Study the drawing (mm; zero at the part's minimum x, y, z) and answer. A direction names the side the tool comes from. Round coordinates to 2 decimals unless told otherwise and drop trailing zeros. Write each loop counter-clockwise with the first axis right and the second up, starting at its lowest first coordinate (ties: lowest second). Pieces come first, ordered by that corner, then holes. Notation, with made-up numbers: M -11.5,14.5 L -1.5,14.5 A18 ccw -1.5,26.5 Z; hole C 61.25,5.5 d5. An arc over 180 degrees is marked long. Write each question's results on one line, items separated by ' | '.
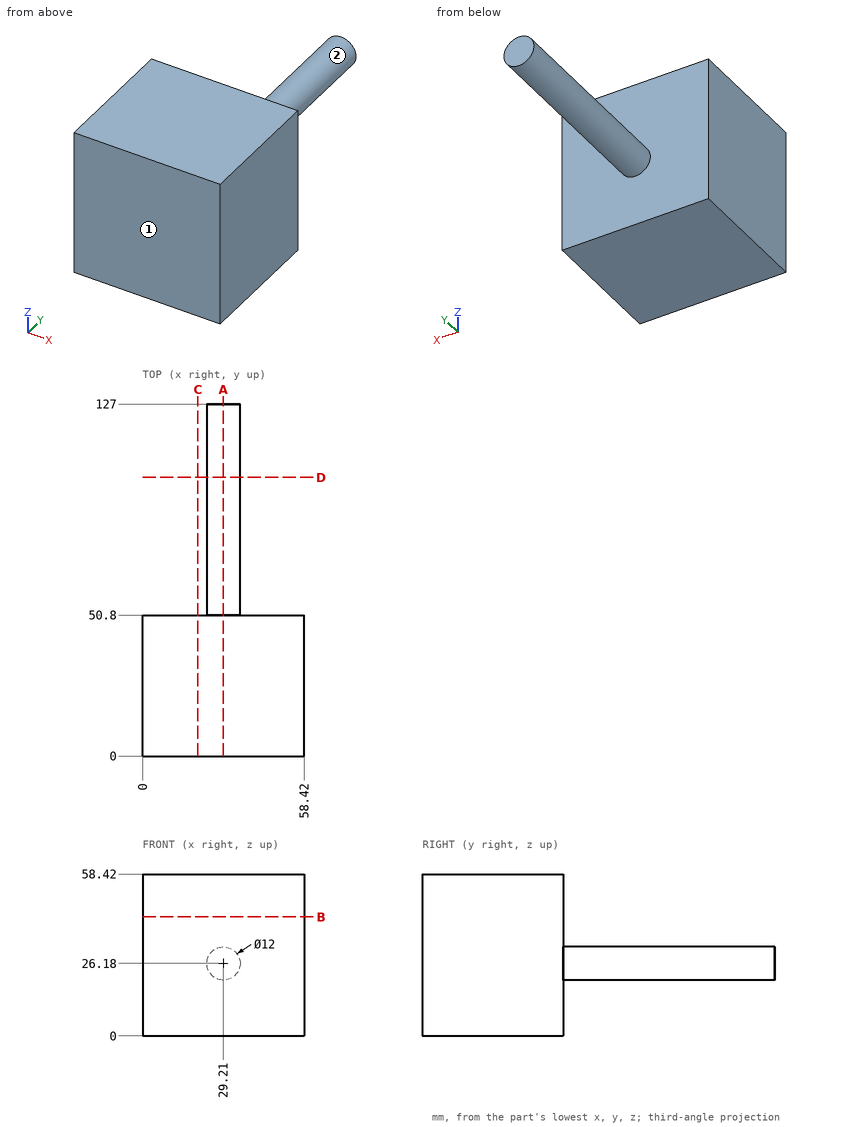
1) Each of these flat-tipped pins is pushed along its axis until it touches: pin 1 (12 mm diameter, centred on x = 21, y = 87.5, fed in from +Z); pin 2 (10 mm diameter, centred on x = 23, z = 49.5, fed in from +Y); pin 3 (3 mm diameter, centred on x = 29, y = 86, fed in from +Z). Where does it stop, or does it pass through?
Return value:
pin 1: z = 31.76 | pin 2: y = 50.8 | pin 3: z = 32.18
2) Section C-C (x = 20) is taken. Determine the outline of the cut face in (y, z).
Return value:
outline: M 0,0 L 50.8,0 L 50.8,58.42 L 0,58.42 Z
3) Section B-B (z = 43) is taken. Determine the outline of the cut face in (x, y).
Return value:
outline: M 0,0 L 58.42,0 L 58.42,50.8 L 0,50.8 Z
4) Section D-D (y = 100.5) is taken. Determine the outline of the cut face in (x, z), then the cut area to 3 significant figures.
Return value:
outline: C 29.21,26.18 d12 | area: 113 mm²
5) A tool of negligible diameter and unlimited length cuts with its end or side. For the marked faces 1 and 2, from which of +Z, -Z, +X, -X, +Y, -Y can it reach the whole face along a straight path? Write none if from no direction.
Return value:
face 1: +Z, -Z, +X, -X, -Y | face 2: +Y
6) Section A-A (x = 29.21) is taken. Determine the outline of the cut face in (y, z), then the cut area to 3 significant figures.
Return value:
outline: M 0,0 L 50.8,0 L 50.8,20.18 L 127,20.18 L 127,32.18 L 50.8,32.18 L 50.8,58.42 L 0,58.42 Z | area: 3,880 mm²
7) Find the intervals of material crossed by line 1 (Y direction, x = 54, z = 13); line 2 (X direction, y = 87.5, z = 28); line 3 (Z direction, x = 28, y = 82.5), in increasing order.
Return value:
line 1: 0 to 50.8 | line 2: 23.49 to 34.93 | line 3: 20.3 to 32.06
